from build123d import *

# Parameters (mm, degrees)
F0_R     = 12
F1_DEPTH = 8
F2_R     = 10.75
F3_DEPTH = 7
F4_W     = 11.5
F4_H     = 12.5
F5_DEPTH = 0.85
F6_R     = 4.148405
F7_DEPTH = 0.15
F8_R     = 0.5


with BuildPart() as f1:
    # F0 (on Top) → F1 (new body)
    with BuildSketch(Plane.XY):
        Circle(F0_R)
    extrude(amount=F1_DEPTH)

    # F2 (on face) → F3 (cut)
    with BuildSketch(Plane(origin=(0, 0, 0), x_dir=(1, 0, 0), z_dir=(0, 0, -1))):
        Circle(F2_R)
    extrude(amount=-F3_DEPTH, mode=Mode.SUBTRACT)

    # F4 (on face) → F5 (cut)
    with BuildSketch(Plane.XY.offset(8)):
        with Locations((-0.252232, 0.222986)):
            Rectangle(F4_W, F4_H)
    extrude(amount=-F5_DEPTH, mode=Mode.SUBTRACT)

    # F6 (on face) → F7 (cut)
    with BuildSketch(Plane.XY.offset(7.15)):
        Circle(F6_R)
    extrude(amount=-F7_DEPTH, mode=Mode.SUBTRACT)

    # F8
    f8_edges = [f1.edges().sort_by_distance(p)[0] for p in [
        (-12, 0, 0),
        (-10.75, 0, 0),
    ]]
    fillet(f8_edges, radius=F8_R)


solid = f1.part
Model file for the job. Use its own axes, mm. A direction names the side the tool comes from. Round coordinates to 2 decimals unless told otherwise and drop trailing zeros. Order: outer loops, then holes, each group sorted by start corner. A loop starts at its lowest first (then second) coordinate and runs counter-clockwise, first axis right, second up.
(1) Pull direction Y, two halves, no side cores. Call faces 1 (the face through (5, 0, 7)), 2 (the face through (0, -8, 8)), 3 (the face through (-11.99, 0.53, 4.2)): released by +Y, released by -Y, zero draft, split by the parting line, or undercut.
(2) Band-saw the part on B-B (y = 0). List the corners of the cut face in (x, z).
(3) Drill centre lines: line 1 (Z direction, x = 10.5, y = 1); line 2 (Z direction, x = 0.75, y = 5.75); line 3 (X direction, y = 2.75, z = 4.25). Where is each one in solid material? Low to high.
(4) 3-axis set-ups, long thin cutter, end or side, ignore diameter. For faces 4 (the face through (-1.4, -10.66, 3.7)), 5 (the face through (-0.3, -6.027, 7.6)): which of +Z, -Z, +X, -X, +Y, -Y reach the whole face in a straight line?
(5) Band-saw the part on A-A (x = 0). List the corners of the cut face in (y, z).
(6) Pin check, flat tips, straight feed: pin 1 (3 mm diameter, centred on y = 8.5, z = 3, fed in from +X); pin 2 (6 mm diameter, centred on x = 5, y = 1.5, fed in from -Z); pin 3 (1.5 mm diameter, centred on x = 2.5, z = 3.5, fed in from +Y); pin 4 (3.5 mm diameter, centred on x = -1, y = 0.5, fed in from +Z). Stop position of each tip, or through.
(7) Band-saw the part on C-C (z = 1.25). List the corners of the cut face in (x, y), then the cut area to 3 significant figures.
Verdict:
1. face 1: undercut
1. face 2: zero draft
1. face 3: split by the parting line
2. outline: (-12, 0.5) arc R0.5 ccw to (-11.5, 0) - (-11.25, 0) arc R0.5 ccw to (-10.75, 0.5) - (-10.75, 7) - (-4.15, 7) - (-4.15, 7.15) - (-6, 7.15) - (-6, 8) - (-12, 8) - close; (4.15, 7) - (10.75, 7) - (10.75, 0.5) arc R0.5 ccw to (11.25, 0) - (11.5, 0) arc R0.5 ccw to (12, 0.5) - (12, 8) - (5.5, 8) - (5.5, 7.15) - (4.15, 7.15) - close
3. line 1: z = 7 to 8
3. line 2: z = 7 to 7.15
3. line 3: x = -11.68 to -10.39, 10.39 to 11.68
4. face 4: -Z
4. face 5: +Z
5. outline: (-12, 0.5) arc R0.5 ccw to (-11.5, 0) - (-11.25, 0) arc R0.5 ccw to (-10.75, 0.5) - (-10.75, 7) - (-4.15, 7) - (-4.15, 7.15) - (-6.03, 7.15) - (-6.03, 8) - (-12, 8) - close; (4.15, 7) - (10.75, 7) - (10.75, 0.5) arc R0.5 ccw to (11.25, 0) - (11.5, 0) arc R0.5 ccw to (12, 0.5) - (12, 8) - (6.47, 8) - (6.47, 7.15) - (4.15, 7.15) - close
6. pin 1: stops at x = 9.75
6. pin 2: stops at z = 7
6. pin 3: stops at y = 11.87
6. pin 4: passes through
7. outline: circle Ø24 at (0, 0); hole circle Ø21.5 at (0, 0)
7. area: 89.3 mm2
